Could you check a few things on this model? Use its own coordinates, in mm. A direction names the side the tool comes from. Give positions to 0.01 mm unless a question says otherwise; leave off trailing zeros. Loops run counter-clockwise (first coordinate to the right, second up) from the corner with the lowest first, then second, coordinate; pieces in that order, holes last. Notation, with made-up numbers: (41, -25.75) - (45, -25.75) arc R23 cw to (45, -11.75) - close; hole circle Ø3 at (-0.5, -4.5). An arc over 180 degrees is marked (long way). One line per item, written item: value. Start each with the question number.
Q1. If we mould it in two halves opening along X, with no side actions, what happens to faces 1 (the face through (-0.86, -25.87, -6.25)), 2 (the face through (15.738, -4.956, -52.493)), 3 (the face through (-6.439, -10.947, -28.382)), 4 (the face through (0, 19, -10))? For each: released by +X, released by -X, zero draft, split by the parting line, or undercut.
Q2. I'm going to push flat-ended pins straight in: P1, Ø6, axis at x = -10.5, y = 4.5, coming from the +Z side; P2, Ø11.5, axis at y = 1, z = -25.5, coming from the +X side; P3, Ø4, axis at y = -8.5, z = -15, coming from the -X side; P4, Ø10, axis at x = -2, z = -22, coming from the +Y side. Where does each tip first touch, or does it pass through?
Q3. For faces 5 (the face through (6.4, 15.4, -53)), 6 (the face through (-6.26, 11.05, -28.38)), 7 (the face through (-4, 17, -31)), which set-ups out of +Z, -Z, +X, -X, +Y, -Y let a thin tool reach every point of the face, with its end or its side?
Q4. If I drill on line 1 (Y direction, x = 0, z = -25); line 2 (X direction, y = 0.5, z = -13); line 3 (X direction, y = -6.5, z = -7.5), over which ranges is the centre line in solid material (lowest first)? Write a range as from..to.
Q5. I want a section at D-D (y = -23.5). Please give me the cut outline in (x, z), then the cut area to 3 significant figures.
Q6. I want a section at A-A (z = -43). Please give me the cut outline in (x, y) (1 decimal).
Q7. I want a section at B-B (y = 0). Please give me the cut outline in (x, z), then the cut area to 3 significant figures.
Q8. I want a section at C-C (y = 9). Count the separate pieces of the cut face and the enclosed holes in it, then the cut area to 3 significant figures.
```python
from build123d import *

# Parameters (mm, degrees)
SKETCH2_R          = 3.96875
CUT_EXTRUDE1_DEPTH = 69.062067304
SKETCH4_W          = 91.060119334
SKETCH4_H          = 85.338920038
CUT_EXTRUDE2_DEPTH = 10
SKETCH5_W          = 59.127494052
SKETCH5_H          = 59.423778288
CUT_EXTRUDE3_DEPTH = 2.5


with BuildPart() as part:
    # Sketch1 → Revolve1 (revolve)
    with BuildSketch(Plane(origin=(0, 0, 0), x_dir=(0, 0, -1), z_dir=(1, 0, 0)), mode=Mode.PRIVATE) as revolve1_sk:
        with BuildLine():
            Line((0, 27.35), (0, 0))
            Line((0, 0), (55, 0))
            Line((55, 0), (55, 15.4625))
            ThreePointArc((55, 15.4625), (54.414213562, 16.876713562), (53, 17.4625))
            Line((53, 17.4625), (53, 16.5))
            Line((53, 16.5), (52, 16.5))
            Line((52, 16.5), (52, 17.4625))
            Line((52, 17.4625), (11, 17.4625))
            ThreePointArc((11, 17.4625), (10.292893219, 17.755393219), (10, 18.4625))
            Line((10, 18.4625), (10, 27.35))
            ThreePointArc((10, 27.35), (9.707106781, 28.057106781), (9, 28.35))
            Line((9, 28.35), (1, 28.35))
            ThreePointArc((1, 28.35), (0.292893219, 28.057106781), (0, 27.35))
        make_face()
    revolve(revolve1_sk.sketch.rotate(Axis((0, 0, 0), (0, 0, -1)), 90), axis=Axis((0, 0, 0), (0, 0, -1)))

    # Sketch2 → Cut-Extrude1 (cut, through all)
    with BuildSketch(Plane.XY):
        with Locations((-19.05, 10.998522628)):
            Circle(SKETCH2_R)
        with Locations((19.05, 10.998522628)):
            Circle(SKETCH2_R)
        with Locations((0, -21.997045256)):
            Circle(SKETCH2_R)
        Polygon((0, 14.664696837), (-12.7, 7.332348419), (-12.7, -7.332348419), (0, -14.664696837), (12.7, -7.332348419), (12.7, 7.332348419), align=None)
    extrude(amount=-CUT_EXTRUDE1_DEPTH, mode=Mode.SUBTRACT)

    # Sketch3 → Cut-Revolve2 (revolve, cut)
    with BuildSketch(Plane(origin=(0, 0, 0), x_dir=(0, 0, -1), z_dir=(1, 0, 0))):
        Polygon((0, 14.664696837), (0, 11.164696837), (3.5, 11.164696837), align=None)
        Polygon((51.5, 11.164696837), (55, 11.164696837), (55, 14.664696837), align=None)
    revolve(axis=Axis((0, 0, -55), (0, 0, 1)), mode=Mode.SUBTRACT)

    # Sketch4 → Cut-Extrude2 (cut)
    with BuildSketch(Plane(origin=(0, 0, -10), x_dir=(-1, 0, 0), z_dir=(0, 0, -1))):
        Rectangle(SKETCH4_W, SKETCH4_H)
        Polygon((0, -39), (33.774990748, 19.5), (-33.774990748, 19.5), align=None, mode=Mode.SUBTRACT)
    extrude(amount=-CUT_EXTRUDE2_DEPTH, mode=Mode.SUBTRACT)

    # Sketch5 → Cut-Extrude3 (cut)
    with BuildSketch(Plane.XY):
        Rectangle(SKETCH5_W, SKETCH5_H)
    extrude(amount=-CUT_EXTRUDE3_DEPTH, mode=Mode.SUBTRACT)


solid = part.part
```
Worked answers:
1. face 1: undercut
1. face 2: split by the parting line
1. face 3: undercut
1. face 4: zero draft
2. P1: stops at z = -2.5
2. P2: stops at x = 17.46
2. P3: stops at x = -16.21
2. P4: stops at y = 17.46
3. face 5: none
3. face 6: +Z, -Z
3. face 7: -Z
4. line 1: y = -17.46..-14.66, 14.66..17.46
4. line 2: x = -17.46..-12.7, 12.7..17.46
4. line 3: x = -18.76..-12.7, 12.7..18.76
5. outline: (-8.95, -10) - (-3.67, -10) - (-3.67, -2.5) - (-8.95, -2.5) - close; (3.67, -10) - (8.95, -10) - (8.95, -2.5) - (3.67, -2.5) - close
5. area: 79.1 mm²
6. outline: circle Ø34.9 at (0, 0); hole (-12.7, -7.3) - (0, -14.7) - (12.7, -7.3) - (12.7, 7.3) - (0, 14.7) - (-12.7, 7.3) - close
7. outline: (-22.52, -10) - (-18.46, -10) arc R1 cw to (-17.46, -11) - (-17.46, -52) - (-16.5, -52) - (-16.5, -53) - (-17.46, -53) arc R2 ccw to (-15.46, -55) - (-14.66, -55) - (-12.7, -53.04) - (-12.7, -2.5) - (-22.52, -2.5) - close; (12.7, -53.04) - (14.66, -55) - (15.46, -55) arc R2 ccw to (17.46, -53) - (16.5, -53) - (16.5, -52) - (17.46, -52) - (17.46, -11) arc R1 cw to (18.46, -10) - (22.52, -10) - (22.52, -2.5) - (12.7, -2.5) - close
7. area: 569 mm²
8. separate pieces: 4
8. enclosed holes: 0
8. area: 610 mm²
